Can you work these out from the model? Positions are in its coordinate system, mm. Face numbers are marked on the shaded views. A direction names the side the tool comes from. Give positions to 0.01 mm unless a question says otherwise; leave off trailing zeros. Loops run counter-clockwise (first coordinate to the right, second up) from the corner with the lowest first, then second, coordinate; pieces in that order, holes last. Notation, with made-up numbers: M -32.5,27.5 L -3.5,27.5 A28 cw -3.5,47.5 Z; hole C -6.5,87 d5. An arc over 180 degrees is marked long. Use CSV: the item, a comma, the result in double quotes.
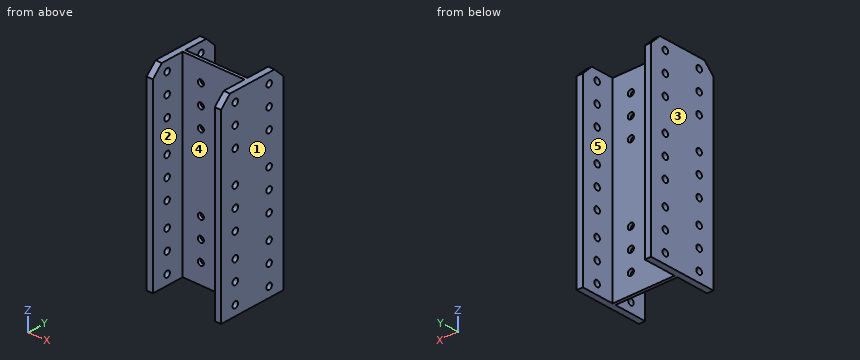
from build123d import *

# Parameters (mm, degrees)
EXTRUDE_1_DEPTH     = 980
SKETCH_2_R          = 15.5
CUT_EXTRUDE_2_DEPTH = 1066.563231348
SKETCH_3_R          = 15.5
CUT_EXTRUDE_3_DEPTH = 1015.883737184
CUT_EXTRUDE_4_DEPTH = 1066.563231348


with BuildPart() as part:
    # 草图1 → 拉伸1 (new body)
    with BuildSketch(Plane.XY):
        Polygon((-158, 175), (-190, 175), (-190, -175), (-158, -175), (-158, -8), (158, -8), (158, -175), (190, -175), (190, 175), (158, 175), (158, 8), (-158, 8), align=None)
    extrude(amount=EXTRUDE_1_DEPTH)

    # 草图2 → 拉伸2 (cut, through all)
    with BuildSketch(Plane(origin=(190, 0, 0), x_dir=(0, 0, -1), z_dir=(1, 0, 0))):
        with Locations(Location((-930, 95, 0), (0, 0, 90))):
            Circle(SKETCH_2_R)
        with Locations(Location((-830, 95, 0), (0, 0, 90))):
            Circle(SKETCH_2_R)
        with Locations(Location((-730, 95, 0), (0, 0, 90))):
            Circle(SKETCH_2_R)
        with Locations(Location((-930, -95, 0), (0, 0, 90))):
            Circle(SKETCH_2_R)
        with Locations(Location((-830, -95, 0), (0, 0, 90))):
            Circle(SKETCH_2_R)
        with Locations(Location((-730, -95, 0), (0, 0, 90))):
            Circle(SKETCH_2_R)
        with Locations(Location((-570, 95, 0), (0, 0, 90))):
            Circle(SKETCH_2_R)
        with Locations(Location((-470, 95, 0), (0, 0, 90))):
            Circle(SKETCH_2_R)
        with Locations(Location((-370, 95, 0), (0, 0, 90))):
            Circle(SKETCH_2_R)
        with Locations(Location((-370, -95, 0), (0, 0, 90))):
            Circle(SKETCH_2_R)
        with Locations(Location((-470, -95, 0), (0, 0, 90))):
            Circle(SKETCH_2_R)
        with Locations(Location((-570, -95, 0), (0, 0, 90))):
            Circle(SKETCH_2_R)
        with Locations(Location((-50, 95, 0), (0, 0, 90))):
            Circle(SKETCH_2_R)
        with Locations(Location((-150, 95, 0), (0, 0, 90))):
            Circle(SKETCH_2_R)
        with Locations(Location((-250, 95, 0), (0, 0, 90))):
            Circle(SKETCH_2_R)
        with Locations(Location((-250, -95, 0), (0, 0, 90))):
            Circle(SKETCH_2_R)
        with Locations(Location((-150, -95, 0), (0, 0, 90))):
            Circle(SKETCH_2_R)
        with Locations(Location((-50, -95, 0), (0, 0, 90))):
            Circle(SKETCH_2_R)
    extrude(amount=-CUT_EXTRUDE_2_DEPTH, mode=Mode.SUBTRACT)

    # 草图3 → 拉伸3 (cut, through all)
    with BuildSketch(Plane(origin=(0, 8, 0), x_dir=(1, 0, 0), z_dir=(0, 1, 0))):
        with Locations(Location((65, -100, 0), (0, 0, 270))):
            Circle(SKETCH_3_R)
        with Locations(Location((-65, -100, 0), (0, 0, 270))):
            Circle(SKETCH_3_R)
        with Locations(Location((65, -200, 0), (0, 0, 270))):
            Circle(SKETCH_3_R)
        with Locations(Location((-65, -200, 0), (0, 0, 270))):
            Circle(SKETCH_3_R)
        with Locations(Location((65, -300, 0), (0, 0, 270))):
            Circle(SKETCH_3_R)
        with Locations(Location((-65, -300, 0), (0, 0, 270))):
            Circle(SKETCH_3_R)
        with Locations(Location((-65, -680, 0), (0, 0, 270))):
            Circle(SKETCH_3_R)
        with Locations(Location((-65, -780, 0), (0, 0, 270))):
            Circle(SKETCH_3_R)
        with Locations(Location((65, -780, 0), (0, 0, 270))):
            Circle(SKETCH_3_R)
        with Locations(Location((65, -880, 0), (0, 0, 270))):
            Circle(SKETCH_3_R)
        with Locations(Location((-65, -880, 0), (0, 0, 270))):
            Circle(SKETCH_3_R)
        with Locations(Location((65, -680, 0), (0, 0, 270))):
            Circle(SKETCH_3_R)
    extrude(amount=-CUT_EXTRUDE_3_DEPTH, mode=Mode.SUBTRACT)

    # 草图4 → 拉伸4 (cut, through all)
    with BuildSketch(Plane(origin=(190, 0, 0), x_dir=(0, 0, -1), z_dir=(1, 0, 0))):
        Polygon((-930, 175), (-980, 125), (-980, 175), align=None)
        Polygon((-980, -125), (-930, -175), (-980, -175), align=None)
    extrude(amount=-CUT_EXTRUDE_4_DEPTH, mode=Mode.SUBTRACT)


solid = part.part
Q1. If we mould it in two halves opening along X, with no side actions, what happens to the marked faces 1, 2 and 3? For each: released by +X, released by -X, zero draft, split by the parting line, or undercut.
Model answer:
face 1,"released by +X"
face 2,"undercut"
face 3,"released by -X"
Q2. Please list where these lines run through material, in increasing order: L1, parallel to X at y = 2, z = 300; L2, parallel to X at y = -114.5, z = 99; L3, parallel to Y at x = 127, z = 451. Write a range as from..to.
Model answer:
L1,"-190..-80.5, -49.5..49.5, 80.5..190"
L2,"-190..-158, 158..190"
L3,"-8..8"
Q3. For the marked faces 4 and 5, which set-ups out of +Z, -Z, +X, -X, +Y, -Y let a thin tool reach every point of the face, with its end or its side?
Model answer:
face 4,"+Z, -Z, -Y"
face 5,"+Z, -Z, +Y"
Q4. I want a section at A-A, the plane y = 52. Please give me the cut outline in (x, z).
Model answer:
outline,"M -190,0 L -158,0 L -158,980 L -190,980 Z; M 158,0 L 190,0 L 190,980 L 158,980 Z"
Q5. I want a section at B-B, the plane z = 570. Please give me the cut outline in (x, y), then the cut area to 3 significant figures.
Model answer:
outline,"M -190,-175 L -158,-175 L -158,-110.5 L -190,-110.5 Z; M -190,-79.5 L -158,-79.5 L -158,-8 L 158,-8 L 158,-79.5 L 190,-79.5 L 190,79.5 L 158,79.5 L 158,8 L -158,8 L -158,79.5 L -190,79.5 Z; M -190,110.5 L -158,110.5 L -158,175 L -190,175 Z; M 158,-175 L 190,-175 L 190,-110.5 L 158,-110.5 Z; M 158,110.5 L 190,110.5 L 190,175 L 158,175 Z"
area,"23,500 mm2"
Q6. I want a section at C-C, the plane z = 300. Please give me the cut outline in (x, y), then the cut area to 3 significant figures.
Model answer:
outline,"M -190,-175 L -158,-175 L -158,-8 L -80.5,-8 L -80.5,8 L -158,8 L -158,175 L -190,175 Z; M -49.5,-8 L 49.5,-8 L 49.5,8 L -49.5,8 Z; M 80.5,-8 L 158,-8 L 158,-175 L 190,-175 L 190,175 L 158,175 L 158,8 L 80.5,8 Z"
area,"26,500 mm2"
Q7. I'm going to push flat-ended pins straight in: P1, Ø8, axis at x = 107.5, z = 268, coming from the +Y side; P2, Ø5, axis at x = 5.5, z = 792, coming from the -Y side. Where does each tip first touch, or does it pass through?
Model answer:
P1,"y = 8"
P2,"y = -8"
Q8. I want a section at D-D, the plane y = -95. State how many separate pieces and enclosed holes the cut face has, then the cut area to 3 significant figures.
Model answer:
separate pieces,"20"
enclosed holes,"0"
area,"44,900 mm2"
